CAD build for the part. Positions are in the model's coordinates, mm. Face numbers are marked on the shaded views. A direction names the side the tool comes from. Give positions to 0.01 mm unless a question says otherwise; leave off trailing zeros. Write each loop counter-clockwise with the first axis right and the second up, starting at its lowest first coordinate (ties: lowest second). Pieces come first, ordered by that corner, then holes. Notation, with made-up numbers: (-19.75, 36) - (15.25, 36) arc R16 cw to (15.25, 61) - close; hole circle Ø4 at (62, 86.25). An arc over 180 degrees is marked (long way). Write item = value, one per line. Start each with the question number.
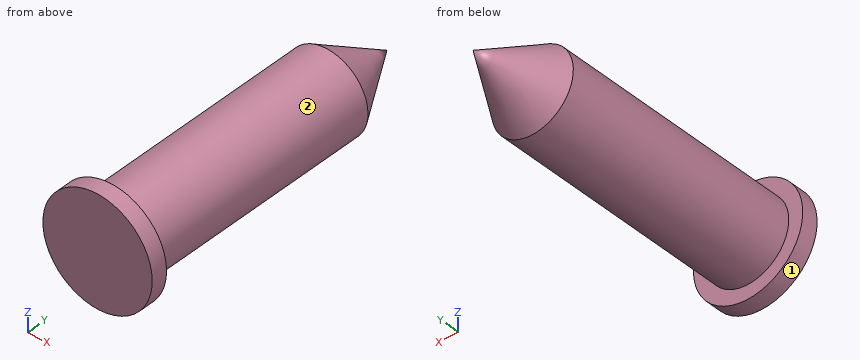
```python
from build123d import *

# Parameters (mm, degrees)
SKETCH1_W           = 5
SKETCH1_H           = 30
SKETCH3_R           = 6.721759799
BOSS_EXTRUDE1_DEPTH = 2


with BuildPart() as part:
    # Sketch1 → Revolve1 (revolve)
    with BuildSketch(Plane(origin=(0, 0, 0), x_dir=(0, 0, -1), z_dir=(1, 0, 0))):
        with Locations((-25.408302522, 49.690625)):
            Rectangle(SKETCH1_W, SKETCH1_H)
    revolve(axis=Axis((0, 64.690625, 22.908302522), (0, -1, 0)))

    # Sketch2 → Revolve5 (revolve)
    with BuildSketch(Plane(origin=(0, 0, 0), x_dir=(0, 0, -1), z_dir=(1, 0, 0))):
        Polygon((-27.908302522, 64.690625), (-22.908302522, 72.998720515), (-22.908302522, 64.690625), align=None)
    revolve(axis=Axis((0, 72.998720515, 22.908302522), (0, -1, 0)))

    # Sketch3 → Boss-Extrude1 (add)
    with BuildSketch(Plane.XZ.offset(-34.690625)):
        with Locations((0, 22.908302522)):
            Circle(SKETCH3_R)
    extrude(amount=BOSS_EXTRUDE1_DEPTH)


solid = part.part
```
1. Tool access for the marked faces 1 and 2: list every direction of +Z, -Z, +X, -X, +Y, -Y with a clear straight run to the whole face (end or side of a thin tool).
2. Pin check, flat tips, straight feed: pin 1 Ø5 at (x, y) = (-1, 51) entering from +Z; pin 2 Ø3 at (y, z) = (39.5, 27) entering from +X; pin 3 Ø2 at (y, z) = (50.5, 18) entering from +X. Stop position of each tip, or through.
3. Cut at A-A (y = 46.5). Give the cut face in (x, z).
4. Wall check: line 1 along X through (y, z) = (46.5, 23); line 2 along Y through (x, z) = (-1.5, 17.5); line 3 along Y through (x, z) = (4, 25.25). Give the ranges that are in metal, low to high.
5. Cut at B-B (z = 17.25). Give the cut face in (x, y), then the cut area to 3 significant figures.
Output:
q1.face_1 = +Y, -Y
q1.face_2 = +Y
q2.pin_1 = 27.91
q2.pin_2 = 4.28
q2.pin_3 = 3.12
q3.outline = circle Ø10 at (0, 22.91)
q4.line_1 = -5 to 5
q4.line_2 = 32.69 to 34.69
q4.line_3 = 32.69 to 65.3
q5.outline = (-3.63, 32.69) - (3.63, 32.69) - (3.63, 34.69) - (-3.63, 34.69) - close
q5.area = 14.5 mm2
